Check sheet for the drawn part. Datum: minimum x, y, z corner. Units: mm. A direction names the side the tool comes from. Coordinates: 2 decimals unless noted, no trailing zeros. Write each loop counter-clockwise with the first axis right and the second up, starting at its lowest first coordinate (ties: lowest second). Pieces come first, ordered by that corner, then holes. Notation, with made-up numbers: M -32.5,65.25 L -0.5,65.25 A18 ccw -0.5,79.25 Z; hole C 88.5,-21 d1. An arc over 180 degrees is marked long. Answer in a Markdown table with one row per item.
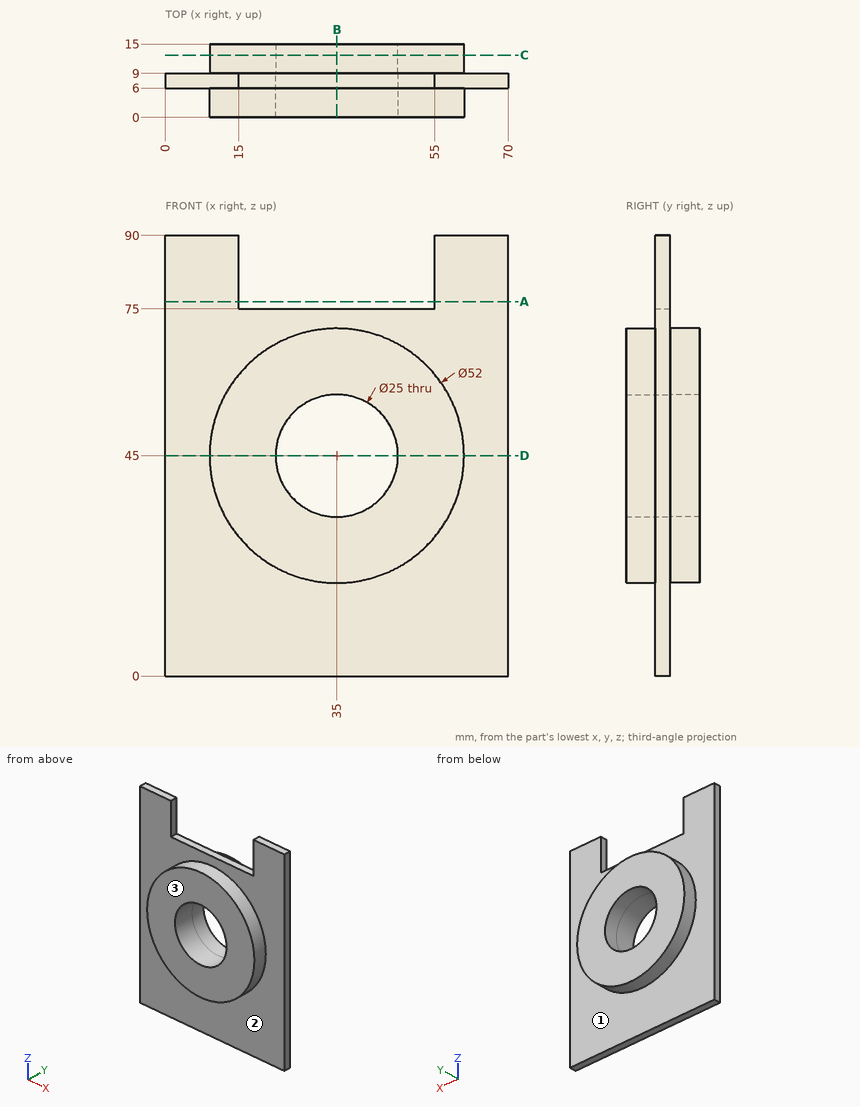
1) Thickness scan on L1, parallel to Z at x = 35, y = 12.3; L2, parallel to Z at x = 35, y = 7; L3, parallel to Y at x = 62.5, z = 38. Record the ranges inside material, lowest first. Write a range as [from, to].
Response values:
| item | result |
|---|---|
| L1 | z = [19, 32.5], [57.5, 71] |
| L2 | z = [0, 32.5], [57.5, 75] |
| L3 | y = [6, 9] |
2) Sectioned sample at C-C (y = 12.75). Record the cut outline in (x, z), then the cut area to 3 significant figures.
Response values:
| item | result |
|---|---|
| outline | C 35,45 d52; hole C 35,45 d25 |
| area | 1,630 mm² |
3) Depth check by flat-ended pin: pin 1 (0.9 mm diameter, centred on x = 36, y = 8, fed in from +Z); pin 2 (3 mm diameter, centred on x = 14.5, z = 26, fed in from -Y). Enter the tip coordinate at first touch or a pass-through.
Response values:
| item | result |
|---|---|
| pin 1 | stops at z = 75 |
| pin 2 | stops at y = 6 |
4) Sectioned sample at B-B (x = 35). Record the cut outline in (y, z).
Response values:
| item | result |
|---|---|
| outline | M 0,19 L 6,19 L 6,0 L 9,0 L 9,19 L 15,19 L 15,32.5 L 0,32.5 Z; M 0,57.5 L 15,57.5 L 15,71 L 9,71 L 9,75 L 6,75 L 6,71 L 0,71 Z |
5) Sectioned sample at A-A (z = 76.5). Record the cut outline in (x, y).
Response values:
| item | result |
|---|---|
| outline | M 0,6 L 15,6 L 15,9 L 0,9 Z; M 55,6 L 70,6 L 70,9 L 55,9 Z |
6) Tool access check on the marked faces 1, 2 and 3. Record the directions out of +Z, -Z, +X, -X, +Y, -Y that give a thin tool (end or side, any length) a straight path to the whole face; none if there is none.
Response values:
| item | result |
|---|---|
| face 1 | +Y |
| face 2 | -Y |
| face 3 | +Z, -Z, +X, -X, -Y |
7) Sectioned sample at D-D (z = 45). Record the cut outline in (x, y), then the cut area to 3 significant figures.
Response values:
| item | result |
|---|---|
| outline | M 0,6 L 9,6 L 9,0 L 22.5,0 L 22.5,15 L 9,15 L 9,9 L 0,9 Z; M 47.5,0 L 61,0 L 61,6 L 70,6 L 70,9 L 61,9 L 61,15 L 47.5,15 Z |
| area | 459 mm² |
